The model under review builds one solid part; all positions refer to its coordinate system, in mm. A direction names the side the tool comes from. Round coordinates to 2 decimals unless told otherwise and drop trailing zeros. Loops run counter-clockwise (first coordinate to the right, second up) from the corner with the lowest first, then second, coordinate; pieces in that order, holes last. Notation, with made-up numbers: M 15.5,48.5 L 73.5,48.5 A24 ccw 73.5,79.5 Z; hole C 66.5,-9 d1. An arc over 180 degrees is marked long. Return JSON: item names as keys, results as strings. Group by question number.
Q1. To check wall thickness, follow line 1 along X through (y, z) = (-0.55, -17); line 2 along Z through (x, y) = (19.5, -0.65); line 3 along X through (y, z) = (-0.95, 8.5). State the ranges of each line that lie inside material, in increasing order.
Q2. Consider section B-B (z = 17). State the section outline as (x, y) points.
Q3. Consider section A-A (x = 0). State the section outline as (y, z) points, and give its area (3 significant figures).
Q4. Consider section C-C (z = 8.5). State the section outline as (x, y) points, and give its area (3 significant figures).
Q5. Consider section D-D (y = 0.5). State the section outline as (x, z) points.
Q6. For faces 4 (the face through (-14.5, 4, 0)), 5 (the face through (18, -1, 17)), 6 (the face through (-15.5, 5, 0)), 7 (the face through (-17, 3, 7.5)), 8 (the face through (-21, 2, 0)), list the 3-axis set-ups (+Z, -Z, +X, -X, +Y, -Y) from which the entire face can be reached by the end or side of a thin tool; tool diameter is ignored.
Q7. Clearance check with flat-ended pins moving along their axes: pin 1 Ø4.5 at (x, z) = (6.01, -6.01) entering from +Y; pin 2 Ø3 at (y, z) = (2.5, 2.5) entering from -X; pin 3 Ø1.6 at (x, z) = (-19.5, -2.5) entering from +Y. State where each tip first meets the part, or that it passes through.
Q8. Draft analysis for pull direction X (two halves, no side actions). For faces 1 (the face through (-16.443, 8, 0)), 2 (the face through (18, -1, -17)), 3 (the face through (-17, 3, -7.5)), state which applies: pulls with the +X half, pulls with the -X half, needs draft (parallel to the pull), parting line crosses it, or undercut.
from build123d import *

# Parameters (mm, degrees)
SKETCH2_W           = 45
SKETCH2_H           = 40
BOSS_EXTRUDE2_DEPTH = 1.5
SKETCH4_R           = 1.4
CUT_EXTRUDE1_DEPTH  = 2.5
SKETCH5_W           = 6.5
SKETCH5_H           = 15
BOSS_EXTRUDE3_DEPTH = 3.5
SKETCH6_W           = 1
SKETCH6_H           = 15
BOSS_EXTRUDE4_DEPTH = 5
BOSS_EXTRUDE5_DEPTH = 15
SKETCH9_R           = 1.5
CUT_EXTRUDE2_DEPTH  = 2.5


with BuildPart() as part:
    # Sketch2 → Boss-Extrude2 (new body)
    with BuildSketch(Plane(origin=(0, 0, 0), x_dir=(1, 0, 0), z_dir=(0, 1, 0))):
        Rectangle(SKETCH2_W, SKETCH2_H)
    extrude(amount=-BOSS_EXTRUDE2_DEPTH)

    # Sketch4 → Cut-Extrude1 (cut, through all)
    with BuildSketch(Plane(origin=(0, 0, 0), x_dir=(1, 0, 0), z_dir=(0, 1, 0))):
        with Locations((0, 8.5)):
            Circle(SKETCH4_R)
        with Locations((6.01040764, 6.01040764)):
            Circle(SKETCH4_R)
        with Locations((0, -8.5)):
            Circle(SKETCH4_R)
        with Locations((-6.01040764, 6.01040764)):
            Circle(SKETCH4_R)
    extrude(amount=-CUT_EXTRUDE1_DEPTH, mode=Mode.SUBTRACT)

    # Sketch5 → Boss-Extrude3 (add)
    with BuildSketch(Plane(origin=(0, 0, 0), x_dir=(1, 0, 0), z_dir=(0, 1, 0))):
        with Locations((-17.75, 0)):
            Rectangle(SKETCH5_W, SKETCH5_H)
    extrude(amount=BOSS_EXTRUDE3_DEPTH)

    # Sketch6 → Boss-Extrude4 (add)
    with BuildSketch(Plane(origin=(0, 3.5, 0), x_dir=(1, 0, 0), z_dir=(0, 1, 0))):
        with Locations((-15, 0)):
            Rectangle(SKETCH6_W, SKETCH6_H)
    extrude(amount=BOSS_EXTRUDE4_DEPTH)

    # Sketch7 → Boss-Extrude5 (add)
    with BuildSketch(Plane.XY.offset(7.5)):
        Polygon((-15.5, 8.5), (-16.442809042, 8.166666667), (-16.442809042, 7.166666667), (-15.5, 6), align=None)
    extrude(amount=-BOSS_EXTRUDE5_DEPTH)

    # Sketch9 → Cut-Extrude2 (cut, through all)
    with BuildSketch(Plane(origin=(0, 0, 0), x_dir=(1, 0, 0), z_dir=(0, 1, 0))):
        with Locations((-12.5, 17)):
            Circle(SKETCH9_R)
        with Locations((-12.5, -17)):
            Circle(SKETCH9_R)
        with Locations((19.5, 17)):
            Circle(SKETCH9_R)
        with Locations((19.5, -17)):
            Circle(SKETCH9_R)
    extrude(amount=-CUT_EXTRUDE2_DEPTH, mode=Mode.SUBTRACT)


solid = part.part
Values:
{
 "1": {"line 1": "x = -22.5 to -14, -11 to 18, 21 to 22.5", "line 2": "z = -20 to -18.5, -15.5 to 15.5, 18.5 to 20", "line 3": "x = -22.5 to -1.4, 1.4 to 22.5"},
 "2": {"outline": "M -22.5,-1.5 L -14,-1.5 L -14,0 L -22.5,0 Z; M -11,-1.5 L 18,-1.5 L 18,0 L -11,0 Z; M 21,-1.5 L 22.5,-1.5 L 22.5,0 L 21,0 Z"},
 "3": {"outline": "M -1.5,-20 L 0,-20 L 0,-9.9 L -1.5,-9.9 Z; M -1.5,-7.1 L 0,-7.1 L 0,7.1 L -1.5,7.1 Z; M -1.5,9.9 L 0,9.9 L 0,20 L -1.5,20 Z", "area": "51.6 mm2"},
 "4": {"outline": "M -22.5,-1.5 L -1.4,-1.5 L -1.4,0 L -22.5,0 Z; M 1.4,-1.5 L 22.5,-1.5 L 22.5,0 L 1.4,0 Z", "area": "63.3 mm2"},
 "5": {"outline": "M -21,-7.5 L -14.5,-7.5 L -14.5,7.5 L -21,7.5 Z"},
 "6": {"face 4": "+Z, -Z, +X, +Y", "face 5": "+Y, -Y", "face 6": "+Z, -Z, -X", "face 7": "+Z, +X, -X, +Y", "face 8": "+Z, -Z, -X, +Y"},
 "7": {"pin 1": "stops at y = 0", "pin 2": "stops at x = -21", "pin 3": "stops at y = 3.5"},
 "8": {"face 1": "pulls with the -X half", "face 2": "undercut", "face 3": "needs draft"}
}
